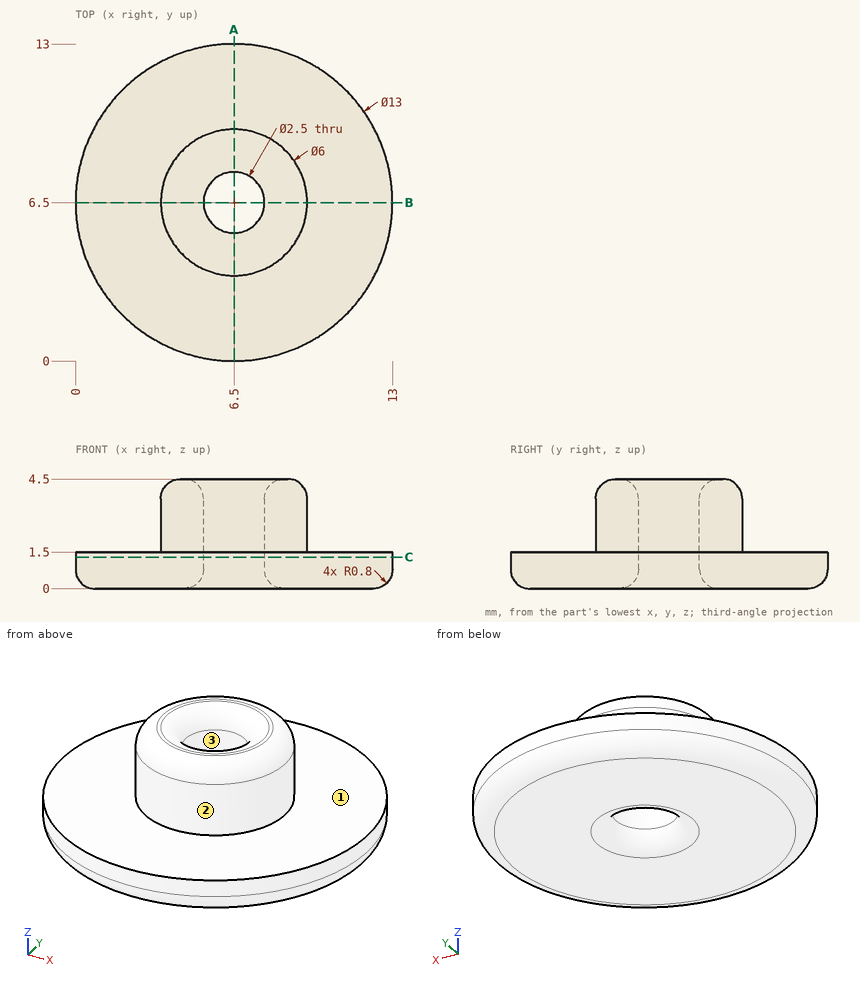
Input: dimensioned drawing with shaded views. Units: mm. Origin: part minimum x, y, z. Round coordinates to 2 decimals unless told otherwise and drop trailing zeros. Loops run counter-clockwise (first coordinate to the right, second up) from the corner with the lowest first, then second, coordinate; pieces in that order, holes last. Notation, with made-up numbers: M -23.75,3 L 30.25,3 A21 cw 30.25,7 Z; hole C 45.5,-3 d11. An arc over 180 degrees is marked long. Answer in a Markdown table with one row per item. Add a question column.
1. Mould query, pull axis X, two halves, no side actions, for the marked faces 1, 2 and 3. Classes: released by +X, released by -X, zero draft, split by the parting line, or undercut.
2. Contact query for flat-ended pins moving along their axis: pin 1 (3 mm diameter, centred on x = 6.5, y = 6.5, fed in from +Z); pin 2 (2 mm diameter, centred on y = 9, z = 3, fed in from +X). Output: stop coordinate, or through.
3. Section C-C (z = 1.3). Output: boundary loops of the cut face in (x, y).
4. Ray query, probe 1 along Z at (x, y) = (3, 4); probe 2 along X at (y, z) = (6, 3.5); probe 3 along X at (y, z) = (7.25, 0.9). Return the intervals inside material, ascending.
5. Section A-A (x = 6.5). Output: boundary loops of the cut face in (y, z).
Values follow:
| question | item | result |
|---|---|---|
| 1 | face 1 | zero draft |
| 1 | face 2 | split by the parting line |
| 1 | face 3 | undercut |
| 2 | pin 1 | z = 4.28 |
| 2 | pin 2 | x = 9.1 |
| 3 | outline | C 6.5,6.5 d13; hole C 6.5,6.5 d2.5 |
| 4 | probe 1 | 0 to 1.5 |
| 4 | probe 2 | 3.54 to 5.35, 7.65 to 9.46 |
| 4 | probe 3 | 0.04 to 5.5, 7.5 to 12.96 |
| 5 | outline | M 0,0.8 A0.8 ccw 0.8,0 L 4.45,0 A0.8 ccw 5.25,0.8 L 5.25,3.7 A0.8 ccw 4.45,4.5 L 4.3,4.5 A0.8 ccw 3.5,3.7 L 3.5,1.5 L 0,1.5 Z; M 7.75,0.8 A0.8 ccw 8.55,0 L 12.2,0 A0.8 ccw 13,0.8 L 13,1.5 L 9.5,1.5 L 9.5,3.7 A0.8 ccw 8.7,4.5 L 8.55,4.5 A0.8 ccw 7.75,3.7 Z |
